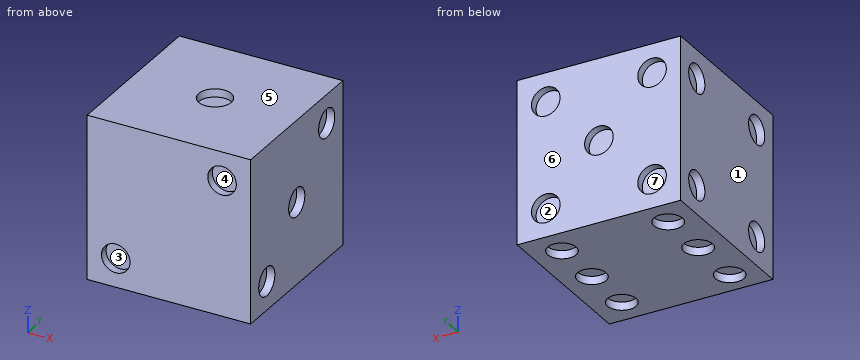
from build123d import *

# Parameters (mm, degrees)
F0_W      = 127
F0_H      = 127
F1_DEPTH  = 127
F2_R      = 12.7
F3_DEPTH  = 6.35
F4_R      = 11.1125
F5_DEPTH  = 6.35
F6_R      = 11.1125
F7_DEPTH  = 6.35
F8_R      = 11.1125
F9_DEPTH  = 6.35
F10_R     = 11.1125
F11_DEPTH = 6.35
F12_R     = 11.1125
F13_DEPTH = 6.35


with BuildPart() as f1:
    # F0 (on Top) → F1 (new body)
    with BuildSketch(Plane.XY):
        with Locations((63.5, 63.5)):
            Rectangle(F0_W, F0_H)
    extrude(amount=F1_DEPTH)

    # F2 (on face) → F3 (cut)
    with BuildSketch(Plane.XY.offset(127)):
        with Locations((63.5, 63.5)):
            Circle(F2_R)
    extrude(amount=-F3_DEPTH, mode=Mode.SUBTRACT)

    # F4 (on face) → F5 (cut)
    with BuildSketch(Plane.XZ):
        with Locations((22.225, 22.225)):
            Circle(F4_R)
        with Locations((104.775, 104.775)):
            Circle(F4_R)
    extrude(amount=-F5_DEPTH, mode=Mode.SUBTRACT)

    # F6 (on face) → F7 (cut)
    with BuildSketch(Plane.YZ.offset(127)):
        with Locations((63.5, 63.5)):
            Circle(F6_R)
        with Locations((22.225, 22.225)):
            Circle(F6_R)
        with Locations((104.775, 104.775)):
            Circle(F6_R)
    extrude(amount=-F7_DEPTH, mode=Mode.SUBTRACT)

    # F8 (on face) → F9 (cut)
    with BuildSketch(Plane(origin=(0, 0, 0), x_dir=(0, -1, 0), z_dir=(-1, 0, 0))):
        with Locations((-104.775, 104.775)):
            Circle(F8_R)
        with Locations((-104.775, 22.225)):
            Circle(F8_R)
        with Locations((-22.225, 104.775)):
            Circle(F8_R)
        with Locations((-22.225, 22.225)):
            Circle(F8_R)
    extrude(amount=-F9_DEPTH, mode=Mode.SUBTRACT)

    # F10 (on face) → F11 (cut)
    with BuildSketch(Plane(origin=(0, 127, 0), x_dir=(-1, 0, 0), z_dir=(0, 1, 0))):
        with Locations((-104.775, 104.775)):
            Circle(F10_R)
        with Locations((-63.5, 63.5)):
            Circle(F10_R)
        with Locations((-22.225, 22.225)):
            Circle(F10_R)
        with Locations((-104.775, 22.225)):
            Circle(F10_R)
        with Locations((-22.225, 104.775)):
            Circle(F10_R)
    extrude(amount=-F11_DEPTH, mode=Mode.SUBTRACT)

    # F12 (on face) → F13 (cut)
    with BuildSketch(Plane(origin=(0, 0, 0), x_dir=(1, 0, 0), z_dir=(0, 0, -1))):
        with Locations((104.775, -104.775)):
            Circle(F12_R)
        with Locations((104.775, -63.5)):
            Circle(F12_R)
        with Locations((104.775, -22.225)):
            Circle(F12_R)
        with Locations((22.225, -63.5)):
            Circle(F12_R)
        with Locations((22.225, -104.775)):
            Circle(F12_R)
        with Locations((22.225, -20.063723)):
            Circle(F12_R)
    extrude(amount=-F13_DEPTH, mode=Mode.SUBTRACT)


solid = f1.part
The listing builds one solid part. Answer for the finished solid, in the listing's coordinates (mm). Face numbers are marked on the shaded views. A direction names the side the tool comes from. Coordinates: 2 decimals unless noted, no trailing zeros. Order: outer loops, then holes, each group sorted by start corner. A loop starts at its lowest first (then second) coordinate and runs counter-clockwise, first axis right, second up. Notation, with made-up numbers: (76.5, -38.75) -> (89.5, -38.75) arc R21 cw to (89.5, -0.75) -> close; hole circle Ø6 at (-7, -5). An arc over 180 degrees is marked (long way). Answer in a Markdown table with one row per item. Add a question column.
Item 1: Find the intervals of material crossed by L1, parallel to X at y = 63.5, z = 4.25; L2, parallel to X at y = 122.5, z = 65; L3, parallel to X at y = 26.5, z = 30, in increasing order. Write a range as from..to.
Item 2: Which of the six approach directions +Z, -Z, +X, -X, +Y, -Y give full straight-line access (tool end or side, diameter ignored) to the marked faces 1, 2 and 3?
Item 3: Each of these flat-tipped pins is pushed along its axis until it touches: P1, Ø11, axis at x = 108.5, y = 107.5, coming from the -Z side; P2, Ø13.5, axis at x = 22.225, z = 22.225, coming from the -Y side; P3, Ø20, axis at y = 22.225, z = 22.225, coming from the +X side. Where does it stop, or does it pass through?
Item 4: Find section A-A (z = 63.5). Write down the section's boundary in (x, y).
Item 5: Find section D-D (z = 17). Write down the section's boundary in (x, y), then the cut area to 3 significant figures.
Item 6: Find section C-C (x = 63.5). Write down the section's boundary in (y, z).
Item 7: Determine the mould class of the marked faces 4, 5, 6 and 7 for opening direction Z: +Z half, -Z half, draft (parallel to the pull), parting line (faces both ways), or undercut.
Item 8: Find section B-B (y = 63.5). Write down the section's boundary in (x, z), then the cut area to 3 significant figures.
Result set:
| question | item | result |
|---|---|---|
| 1 | L1 | x = 0..11.11, 33.34..93.66, 115.89..127 |
| 1 | L2 | x = 0..52.49, 74.51..127 |
| 1 | L3 | x = 6.35..120.65 |
| 2 | face 1 | +Z, -Z, -X, +Y, -Y |
| 2 | face 2 | +Y |
| 2 | face 3 | -Y |
| 3 | P1 | stops at z = 6.35 |
| 3 | P2 | stops at y = 6.35 |
| 3 | P3 | stops at x = 120.65 |
| 4 | outline | (0, 0) -> (127, 0) -> (127, 52.39) -> (120.65, 52.39) -> (120.65, 74.61) -> (127, 74.61) -> (127, 127) -> (74.61, 127) -> (74.61, 120.65) -> (52.39, 120.65) -> (52.39, 127) -> (0, 127) -> close |
| 5 | outline | (0, 0) -> (12.42, 0) -> (12.42, 6.35) -> (32.03, 6.35) -> (32.03, 0) -> (127, 0) -> (127, 12.42) -> (120.65, 12.42) -> (120.65, 32.03) -> (127, 32.03) -> (127, 127) -> (114.58, 127) -> (114.58, 120.65) -> (94.97, 120.65) -> (94.97, 127) -> (32.03, 127) -> (32.03, 120.65) -> (12.42, 120.65) -> (12.42, 127) -> (0, 127) -> (0, 114.58) -> (6.35, 114.58) -> (6.35, 94.97) -> (0, 94.97) -> (0, 32.03) -> (6.35, 32.03) -> (6.35, 12.42) -> (0, 12.42) -> close |
| 5 | area | 15,400 mm² |
| 6 | outline | (0, 0) -> (127, 0) -> (127, 52.39) -> (120.65, 52.39) -> (120.65, 74.61) -> (127, 74.61) -> (127, 127) -> (76.2, 127) -> (76.2, 120.65) -> (50.8, 120.65) -> (50.8, 127) -> (0, 127) -> close |
| 7 | face 4 | undercut |
| 7 | face 5 | +Z half |
| 7 | face 6 | draft |
| 7 | face 7 | undercut |
| 8 | outline | (0, 0) -> (11.11, 0) -> (11.11, 6.35) -> (33.34, 6.35) -> (33.34, 0) -> (93.66, 0) -> (93.66, 6.35) -> (115.89, 6.35) -> (115.89, 0) -> (127, 0) -> (127, 52.39) -> (120.65, 52.39) -> (120.65, 74.61) -> (127, 74.61) -> (127, 127) -> (76.2, 127) -> (76.2, 120.65) -> (50.8, 120.65) -> (50.8, 127) -> (0, 127) -> close |
| 8 | area | 15,500 mm² |
